The listing builds one solid part. Answer for the finished solid, in the listing's coordinates (mm). A direction names the side the tool comes from. Coordinates: 2 decimals unless noted, no trailing zeros. Write each loop counter-clockwise with the first axis right and the second up, starting at its lowest first coordinate (ties: lowest second). Pieces come first, ordered by that corner, then holes. Notation, with made-up numbers: M -22.5,-31.5 L 23.5,-31.5 A23 cw 23.5,-20.5 Z; hole C 51,25.5 d8. An arc over 180 degrees is marked long. Answer as CSV lines item,"result".
Autodesk Fusion 360 part; units mm, degrees
sketch "스케치1" plane through (0, 0, 0) normal (0, 0, 1) x (1, 0, 0)
  line L0 (10, 24) -> (-10, 24)
  line L1 (-10, 24) -> (-10, -24)
  line L2 (-10, -24) -> (10, -24)
  line L3 (10, -24) -> (10, 24)
  line L4 (10, 24) -> (-10, -24) construction
  line L5 (-10, 24) -> (10, -24) construction
  line L6 (0, 0) -> (0, 11)
  circle A0 centre (0, 11) radius 1.6
  line L7 (0, 0) -> (0, -11)
  circle A1 centre (0, -11) radius 1.6
  circle A2 centre (0, 0) radius 2.65
  dimension "d1" = 20
  dimension "d2" = 48
  dimension "d3" = 11
  dimension "d4" = 3.2
  dimension "d5" = 11
  dimension "d6" = 3.2
  dimension "d7" = 5.3
extrude "돌출1" add sketch "스케치1" along normal blind 5
extrude "돌출2" add sketch "스케치1" along normal blind 2.8 contours A0 | A1
Q1. Find section C-C (z = 1.65). Give the vertices of the cut face in (x, y).
Output:
outline,"M -10,-24 L 10,-24 L 10,24 L -10,24 Z; hole C 0,0 d5.3"
Q2. Find section B-B (x = 0). Give the vertices of the cut face in (y, z), and give its area (3 significant figures).
Output:
outline,"M -24,0 L -2.65,0 L -2.65,5 L -9.4,5 L -9.4,2.8 L -12.6,2.8 L -12.6,5 L -24,5 Z; M 2.65,0 L 24,0 L 24,5 L 12.6,5 L 12.6,2.8 L 9.4,2.8 L 9.4,5 L 2.65,5 Z"
area,"199 mm2"
Q3. For faces 5 (the cylindrical face through (-0.35, -9.44, 3.88)), 6 (the flat face through (4, 0, 0)), determine the directions among +Z, -Z, +X, -X, +Y, -Y from which every point of the face is accessible in a straight line to the end or side of a thin tool.
Output:
face 5,"+Z"
face 6,"-Z, +X, -X, +Y, -Y"
Q4. The mould has two halves that part along Y. Classify faces 1 (the flat face through (0, 11, 2.8)), 2 (the cylindrical face through (-0.35, 12.56, 3.88)), 3 (the flat face through (0, 24, 2)), 4 (the flat face through (4, 0, 5)): pulls with the +Y half, pulls with the -Y half, needs draft (parallel to the pull), parting line crosses it, or undercut.
Output:
face 1,"undercut"
face 2,"undercut"
face 3,"pulls with the +Y half"
face 4,"needs draft"
Q5. Find section D-D (y = 11). Give the vertices of the cut face in (x, z).
Output:
outline,"M -10,0 L 10,0 L 10,5 L 1.6,5 L 1.6,2.8 L -1.6,2.8 L -1.6,5 L -10,5 Z"
Q6. A flat-ended cylindrical pin translates along its axis: pin 1 Ø1 at (x, y) = (1, -11) entering from +Z. Find the tip coordinate at first contact, or state that the pin passes through.
Output:
pin 1,"z = 2.8"
Q7. Straight lines are drawn through the part: line 1 (Y direction, x = 0, z = 4.25); line 2 (Y direction, x = 0, z = 1.15); line 3 (X direction, y = -11, z = 4.55). For each, find the intervals that lie inside material, in ascending order.
Output:
line 1,"-24 to -12.6, -9.4 to -2.65, 2.65 to 9.4, 12.6 to 24"
line 2,"-24 to -2.65, 2.65 to 24"
line 3,"-10 to -1.6, 1.6 to 10"
Q8. Find section A-A (y = 0). Give the vertices of the cut face in (x, z).
Output:
outline,"M -10,0 L -2.65,0 L -2.65,5 L -10,5 Z; M 2.65,0 L 10,0 L 10,5 L 2.65,5 Z"
